from build123d import *
from build123d.topology import SkipClean

# Parameters (mm, degrees)
SKETCH1_R           = 3.325
SKETCH1_R_2         = 8.5
BOSS_EXTRUDE1_DEPTH = 2.5
SKETCH2_R           = 70.911866835
SKETCH2_R_2         = 13.5
CUT_EXTRUDE1_DEPTH  = 2.5
SKETCH3_R           = 13.5
SKETCH3_R_2         = 8.5
BOSS_EXTRUDE2_DEPTH = 5
FILLET1_R           = 1.5


with BuildPart() as part:
    # Sketch1 → Boss-Extrude1 (new, symmetric)
    with BuildSketch(Plane.XY):
        with BuildLine():
            ThreePointArc((60.622067271, 14.206532436), (59.125498335, 14.810906809), (57.524692071, 15.016834632))
            Line((57.524692071, 15.016834632), (56.997116089, 14.994793348))
            Line((56.997116089, 14.994793348), (37.942484943, 14.198721238))
            ThreePointArc((37.942484943, 14.198721238), (29.810784304, 16.198484397), (24.018273447, 22.245833067))
            ThreePointArc((24.018273447, 22.245833067), (11.4864831, 29.488233713), (-0.397539124, 21.225779345))
            ThreePointArc((-0.397539124, 21.225779345), (-5.665447564, 14.71634399), (-13.602008261, 12.045274491))
            Line((-13.602008261, 12.045274491), (-32.656639407, 11.249202381))
            ThreePointArc((-32.656639407, 11.249202381), (-35.431571333, 10.60798438), (-37.643867273, 8.81434161))
            ThreePointArc((-37.643867273, 8.81434161), (-38.932803958, 4.139738531), (-36.53293032, -0.073796594))
            Line((-36.53293032, -0.073796594), (10.980057512, -36.923376572))
            ThreePointArc((10.980057512, -36.923376572), (14.305396611, -37.984745832), (17.530617501, -36.649704619))
            Line((17.530617501, -36.649704619), (61.804364137, 4.034578786))
            ThreePointArc((61.804364137, 4.034578786), (63.807395856, 9.422079897), (60.622067271, 14.206532436))
        make_face()
        with Locations((14.093347289, -32.909173442)):
            Circle(SKETCH1_R, mode=Mode.SUBTRACT)
        with BuildLine():
            Line((-19.81205116, 3.778850103), (44.820399723, 6.479090855))
            ThreePointArc((44.820399723, 6.479090855), (47.71753436, 4.629103679), (46.975509685, 1.272730481))
            Line((46.975509685, 1.272730481), (15.799754589, -27.375471944))
            ThreePointArc((15.799754589, -27.375471944), (13.895096583, -28.163882109), (11.93131365, -27.537089238))
            Line((11.93131365, -27.537089238), (-21.525382137, -1.589127566))
            ThreePointArc((-21.525382137, -1.589127566), (-22.544780206, 1.693656197), (-19.81205116, 3.778850103))
        make_face(mode=Mode.SUBTRACT)
        with Locations((-32.656639407, 4.924202381)):
            Circle(SKETCH1_R, mode=Mode.SUBTRACT)
        with Locations((12.05, 16)):
            Circle(SKETCH1_R_2, mode=Mode.SUBTRACT)
        with Locations((57.524692071, 8.691834632)):
            Circle(SKETCH1_R, mode=Mode.SUBTRACT)
    extrude(amount=BOSS_EXTRUDE1_DEPTH, both=True)

    # Sketch2 → Cut-Extrude1 (cut)
    with SkipClean():  # the faces are left unmerged after this step: merging them gives an invalid solid
        with BuildSketch(Plane.XY.offset(2.5)):
            with Locations((12.05, 16)):
                Circle(SKETCH2_R)
            with Locations((12.05, 16)):
                Circle(SKETCH2_R_2, mode=Mode.SUBTRACT)
        extrude(amount=-CUT_EXTRUDE1_DEPTH, mode=Mode.SUBTRACT)

    # Sketch3 → Boss-Extrude2 (add)
    with BuildSketch(Plane.XY.offset(2.5)):
        with Locations(Location((12.05, 16, 0), (0, 0, 157.226152371))):
            Circle(SKETCH3_R)
        with Locations((12.05, 16)):
            Circle(SKETCH3_R_2, mode=Mode.SUBTRACT)
    extrude(amount=-BOSS_EXTRUDE2_DEPTH)

    # Fillet1
    fillet1_edges = [part.edges().sort_by_distance(p)[0] for p in [
        (25.161477635, 19.215455525, 2.5),
    ]]
    fillet(fillet1_edges, radius=FILLET1_R)


solid = part.part
Here's how the part is built. I have some questions about the finished solid (model axes, mm). A direction names the side the tool comes from. Coordinates: 2 decimals unless noted, no trailing zeros. Order: outer loops, then holes, each group sorted by start corner. A loop starts at its lowest first (then second) coordinate and runs counter-clockwise, first axis right, second up. Notation, with made-up numbers: (20, 78.25) -> (66, 78.25) arc R13 cw to (66, 87.25) -> close; hole circle Ø1 at (46, -27). An arc over 180 degrees is marked (long way). Answer in a Markdown table with one row per item.
(1) On a 3-axis mill with a long thin cutter (end or side, diameter ignored), from which of +Z, -Z, +X, -X, +Y, -Y can I reach the whole of each face in a straight line? I mean faces 5 (the face through (29.91, 16.14, -1.23)), 6 (the face through (-22.996, 11.653, -1.232)), 7 (the face through (-22.56, 1.64, -1.23)). Say none if no direction works.
Answer key:
| item | result |
|---|---|
| face 5 | +Z, -Z, +Y |
| face 6 | +Z, -Z, -X, +Y |
| face 7 | +Z, -Z |
(2) I want a section at A-A on x = 27. List the corners of the cut face in (y, z) for me.
Answer key:
| item | result |
|---|---|
| outline | (-27.95, -2.5) -> (-17.08, -2.5) -> (-17.08, 0) -> (-27.95, 0) -> close; (5.73, -2.5) -> (18.3, -2.5) -> (18.3, 0) -> (5.73, 0) -> close |
(3) I want a section at C-C on x = 43. List the corners of the cut face in (y, z) for me, then the cut area to 3 significant figures.
Answer key:
| item | result |
|---|---|
| outline | (-13.25, -2.5) -> (-2.38, -2.5) -> (-2.38, 0) -> (-13.25, 0) -> close; (6.4, -2.5) -> (14.41, -2.5) -> (14.41, 0) -> (6.4, 0) -> close |
| area | 47.2 mm^2 |
(4) Will these pins go through, and if not, where does the flat tip stop? pin 1 Ø4 at (x, y) = (25, 12.5) entering from +Z; pin 2 Ø3 at (y, z) = (-15.5, -2) entering from +X; pin 3 Ø7.5 at (x, y) = (57.52, 8.69) entering from +Z; pin 4 Ø4 at (x, y) = (-32.66, 4.92) entering from -Z.
Answer key:
| item | result |
|---|---|
| pin 1 | z = 2.5 |
| pin 2 | x = 42.18 |
| pin 3 | z = 0 |
| pin 4 | through |
(5) Thinking about a two-plate mould opening in Y: for faces 1 (the face through (15.97, 8.46, -0.04)), 2 (the face through (39.36, -16.59, -1.23)), 3 (the face through (-5.568, 14.785, -1.232)), 4 (the face through (9.2, 24.2, 2.5)), which applies, +Y half, -Y half, draft (parallel to the pull), parting line (faces both ways), or undercut?
Answer key:
| item | result |
|---|---|
| face 1 | undercut |
| face 2 | -Y half |
| face 3 | +Y half |
| face 4 | draft |
(6) I want a section at B-B on z = -1. Count the separate pieces of the cut face and the enclosed holes in it, then the cut area to 3 significant figures.
Answer key:
| item | result |
|---|---|
| separate pieces | 1 |
| enclosed holes | 5 |
| area | 1,920 mm^2 |
(7) Please list where these lines run through material, in increasing order: probe 1 along Z at (x, y) = (54, 1); probe 2 along Y at (x, z) = (8.5, 1.4); probe 3 along X at (y, z) = (18, -0.2).
Answer key:
| item | result |
|---|---|
| probe 1 | -2.5 to 0 |
| probe 2 | 3.03 to 8.28, 23.72 to 28.97 |
| probe 3 | -2.25 to 3.79, 20.31 to 27.32 |
